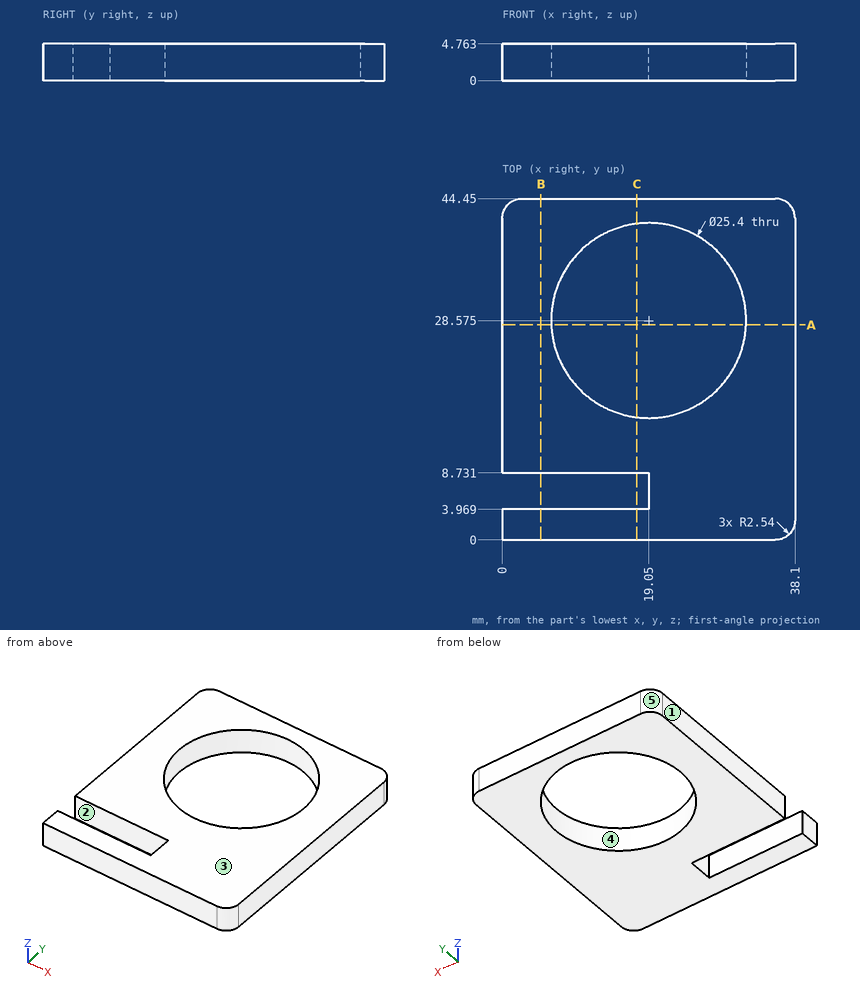
Job drawing, mm, ordinate dimensions from the low corner. One solid piece. A direction names the side the tool comes from. Round coordinates to 2 decimals unless told otherwise and drop trailing zeros. Write each loop counter-clockwise with the first axis right and the second up, starting at its lowest first coordinate (ties: lowest second). Pieces come first, ordered by that corner, then holes.
1) Band-saw the part on B-B, the plane x = 5. List the corners of the cut face in (y, z), and give its area (3 significant figures).
2) Mould opens along Y. For the marked faces 3, 4 and 5 say: +Y half, -Y half, draft (parallel to the pull), parting line (faces both ways), or undercut.
3) Band-saw the part on A-A, the plane y = 28. List the corners of the cut face in (x, z).
4) Drill centre lines: probe 1 along Y at (x, z) = (14.5, 4.35); probe 2 along Y at (x, z) = (6, 3.2); probe 3 along X at (y, z) = (28.5, 4.2). Where is each one in solid material? Low to high.
5) Pin check, flat tips, straight feed: pin 1 (1.4 mm diameter, centred on y = 7, z = 2, fed in from -X); pin 2 (20.5 mm diameter, centred on x = 19.05, y = 28.575, fed in from +Z). Stop position of each tip, or through.
6) Band-saw the part on C-C, the plane x = 17.5. List the corners of the cut face in (y, z).
7) 3-axis set-ups, long thin cutter, end or side, ignore diameter. For the marked faces 1 and 2: which of +Z, -Z, +X, -X, +Y, -Y reach the whole face in a straight line?
Ans:
1. outline: (0, 0) - (3.97, 0) - (3.97, 4.76) - (0, 4.76) - close; (8.73, 0) - (44.45, 0) - (44.45, 4.76) - (8.73, 4.76) - close
1. area: 189 mm2
2. face 3: draft
2. face 4: undercut
2. face 5: +Y half
3. outline: (0, 0) - (6.36, 0) - (6.36, 4.76) - (0, 4.76) - close; (31.74, 0) - (38.1, 0) - (38.1, 4.76) - (31.74, 4.76) - close
4. probe 1: y = 0 to 3.97, 8.73 to 16.72, 40.43 to 44.45
4. probe 2: y = 0 to 3.97, 8.73 to 44.45
4. probe 3: x = 0 to 6.35, 31.75 to 38.1
5. pin 1: stops at x = 19.05
5. pin 2: passes through
6. outline: (0, 0) - (3.97, 0) - (3.97, 4.76) - (0, 4.76) - close; (8.73, 0) - (15.97, 0) - (15.97, 4.76) - (8.73, 4.76) - close; (41.18, 0) - (44.45, 0) - (44.45, 4.76) - (41.18, 4.76) - close
7. face 1: +Z, -Z, -X, +Y, -Y
7. face 2: +Z, -Z, -X
